Can you work these out from the drawing? Everything is in mm from the part's minimum corner. A direction names the side the tool comes from. Coordinates: 2 decimals unless noted, no trailing zeros. Write each loop counter-clockwise with the first axis right and the second up, starting at its lowest first coordinate (ties: lowest second). Pieces come first, ordered by that corner, then holes. Notation, with made-up numbers: (41.5, 52.5) -> (62.5, 52.5) arc R23 ccw to (62.5, 75.5) -> close; hole circle Ø10 at (-31, -5.5). An arc over 180 degrees is marked (long way). Use a Markdown table: item, result. Add a question column.
Item 1: On a 3-axis mill with a long thin cutter (end or side, diameter ignored), from which of +Z, -Z, +X, -X, +Y, -Y can I reach the whole of each face in a straight line? I mean the marked faces 1 and 2. Say none if no direction works.
Item 2: If I drill on line 1 along Y through (x, z) = (6.25, 3); line 2 along X through (y, z) = (64.5, 6); line 3 along X through (y, z) = (24, 14), over which ranges is the centre line in solid material (lowest first)? Write a range as from..to.
Item 3: Imagine slicing it at D-D, the plane z = 28.5. Write out the boundary of the cut face in (x, y), and give its area (3 significant figures).
Item 4: Imagine slicing it at A-A, the plane x = 5.5. Write out the boundary of the cut face in (y, z), and give its area (3 significant figures).
Item 5: Will these pins go through, and if not, where does the flat tip stop? pin 1 Ø4 at (x, z) = (7, 10.5) entering from +Y; pin 2 Ø1.5 at (x, y) = (2.5, 59) entering from +Z; pin 3 Ø1.4 at (x, y) = (10, 10.5) entering from +Z.
Item 6: Imagine slicing it at B-B, the plane z = 8. Write out the boundary of the cut face in (x, y) (1 decimal), and give its area (3 significant figures).
Item 7: Imagine slicing it at C-C, the plane y = 63.5. Write out the boundary of the cut face in (x, z).
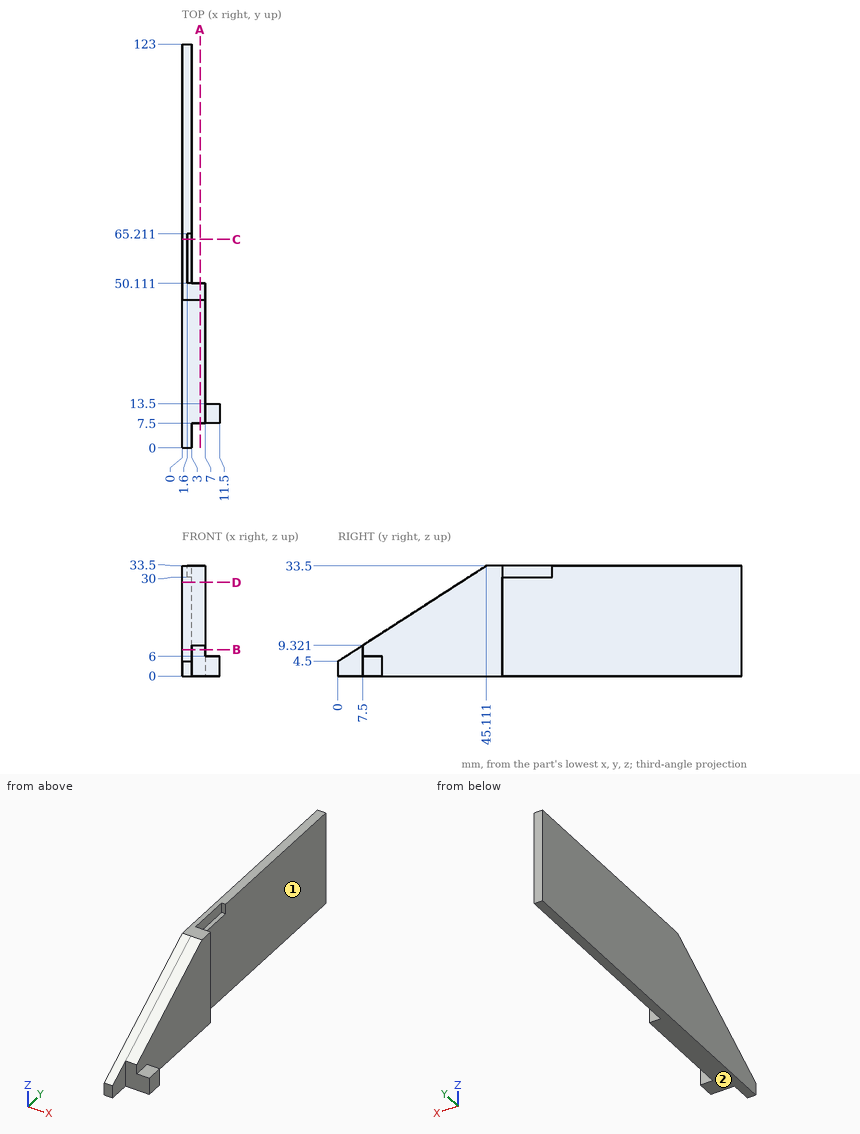
Ans:
| question | item | result |
|---|---|---|
| 1 | face 1 | +Z, -Z, +X, +Y |
| 1 | face 2 | -Z, +X, -X, +Y, -Y |
| 2 | line 1 | y = 7.5..50.11 |
| 2 | line 2 | x = 0..3 |
| 2 | line 3 | x = 0..7 |
| 3 | outline | (0, 37.33) -> (7, 37.33) -> (7, 50.11) -> (3, 50.11) -> (3, 123) -> (0, 123) -> close |
| 3 | area | 308 mm^2 |
| 4 | outline | (7.5, 0) -> (50.11, 0) -> (50.11, 33.5) -> (45.11, 33.5) -> (7.5, 9.32) -> close |
| 4 | area | 973 mm^2 |
| 5 | pin 1 | stops at y = 50.11 |
| 5 | pin 2 | stops at z = 30 |
| 5 | pin 3 | stops at z = 6 |
| 6 | outline | (0, 5.4) -> (3, 5.4) -> (3, 7.5) -> (7, 7.5) -> (7, 50.1) -> (3, 50.1) -> (3, 123) -> (0, 123) -> close |
| 6 | area | 523 mm^2 |
| 7 | outline | (0, 0) -> (3, 0) -> (3, 30) -> (1.6, 30) -> (1.6, 33.5) -> (0, 33.5) -> close |
